from build123d import *

# Parameters (mm, degrees)
F1_DEPTH = 92.5
F2_W     = 220
F2_H     = 175
F3_DEPTH = 200
F4_DEPTH = 195
F5_DEPTH = 2
F6_DEPTH = 2


with BuildPart() as f1:
    # F0 (on Front) → F1 (new body, symmetric)
    with BuildSketch(Plane.XZ):
        with BuildLine():
            Line((-39.8502688743, 141.3978409826), (-105.0004470674, 141.3978409826))
            Line((-105.0004470674, 141.3978409826), (-105.0004470674, -28.6021590174))
            Line((-105.0004470674, -28.6021590174), (124.9995529326, -28.6021590174))
            Line((124.9995529326, -28.6021590174), (124.9995529326, 51.3978409826))
            Line((124.9995529326, 51.3978409826), (0, 134.314134717))
            ThreePointArc((0, 134.314134717), (-19.6127861763, 139.6131417621), (-39.8502688743, 141.3978409826))
        make_face()
    extrude(amount=F1_DEPTH, both=True)

    # F2 (on face) → F3 (join)
    with BuildSketch(Plane(origin=(0, 0, -28.6021590174), x_dir=(1, 0, 0), z_dir=(0, 0, -1))):
        with Locations((9.9995529326, 0)):
            Rectangle(F2_W, F2_H)
    extrude(amount=-F3_DEPTH)

    # F4 (cut): a face of the model
    f4_faces = [f1.faces().sort_by_distance(p)[0] for p in [
        (9.9995529326, 0, 171.3978409826),
    ]]
    extrude(f4_faces, amount=-F4_DEPTH, mode=Mode.SUBTRACT)

    # F5 (add): a face of the model
    f5_faces = [f1.faces().sort_by_distance(p)[0] for p in [
        (-100.0004470674, 0, 58.8978409826),
    ]]
    extrude(f5_faces, amount=F5_DEPTH)

    # F6 (add): a face of the model
    f6_faces = [f1.faces().sort_by_distance(p)[0] for p in [
        (119.9995529326, 0, 15.5561727884),
    ]]
    extrude(f6_faces, amount=F6_DEPTH)


solid = f1.part
The listing builds one solid part. Answer for the finished solid, in the listing's coordinates (mm). A direction names the side the tool comes from. Give positions to 0.01 mm unless a question says otherwise; leave off trailing zeros. Write each loop counter-clockwise with the first axis right and the second up, starting at its lowest first coordinate (ties: lowest second). Pieces come first, ordered by that corner, then holes. Notation, with made-up numbers: (42, 48.25) - (69, 48.25) arc R27 cw to (69, 72.25) - close; hole circle Ø1 at (-19.5, 19). An arc over 180 degrees is marked (long way). Use a Markdown table: item, result.
1. Section A-A on z = 7 is taken. Write down the section's boundary in (x, y), plus the area to 3 significant figures.
Values follow:
| item | result |
|---|---|
| outline | (-105, -92.5) - (125, -92.5) - (125, 92.5) - (-105, 92.5) - close; hole (-98, -87.5) - (118, -87.5) - (118, 87.5) - (-98, 87.5) - close |
| area | 4,750 mm² |
2. Section C-C on y = -6.5 is taken. Write down the section's boundary in (x, z), plus the area to 3 significant figures.
Values follow:
| item | result |
|---|---|
| outline | (-105, -28.6) - (125, -28.6) - (125, 51.4) - (120, 54.71) - (118, 54.71) - (118, -23.6) - (-98, -23.6) - (-98, 141.4) - (-105, 141.4) - close |
| area | 2,840 mm² |
3. A tool of negligible diameter and unlimited length cuts with its end or side. For faces 1 (the flat face through (125, -1, 11)), 2 (the flat face through (8, -1, -23.602)), from which of +Z, -Z, +X, -X, +Y, -Y can it reach the whole face along a straight path? Write none if from no direction.
Values follow:
| item | result |
|---|---|
| face 1 | +Z, -Z, +X, +Y, -Y |
| face 2 | +Z |
4. Section D-D on z = 70 is taken. Write down the section's boundary in (x, y), plus the area to 3 significant figures.
Values follow:
| item | result |
|---|---|
| outline | (-105, -92.5) - (96.96, -92.5) - (96.96, -87.5) - (-98, -87.5) - (-98, 87.5) - (96.96, 87.5) - (96.96, 92.5) - (-105, 92.5) - close |
| area | 3,240 mm² |
5. Each of these flat-tipped pins is pushed along its axis until it touches: P1, Ø0.6, axis at x = 118.5, y = -26, coming from the +Z side; P2, Ø5, axis at x = -65, y = 28.5, coming from the +Z side. Where does it stop, or does it pass through?
Values follow:
| item | result |
|---|---|
| P1 | stops at z = 54.71 |
| P2 | stops at z = -23.6 |
6. For a pull along Y with two mould halves and no side action, classify faces 3 (the flat face through (9, 87.5, 42)), 4 (the flat face through (8, -92.5, 39)), 5 (the flat face through (8, -1, -28.602)) as released by +Y, released by -Y, zero draft, split by the parting line, or undercut.
Values follow:
| item | result |
|---|---|
| face 3 | undercut |
| face 4 | released by -Y |
| face 5 | zero draft |
7. Section B-B on x = -47 is taken. Write down the section's boundary in (y, z).
Values follow:
| item | result |
|---|---|
| outline | (-92.5, -28.6) - (92.5, -28.6) - (92.5, 141.4) - (87.5, 141.4) - (87.5, -23.6) - (-87.5, -23.6) - (-87.5, 141.4) - (-92.5, 141.4) - close |
8. Find the intervals of material crossed by probe 1 along Y at (x, z) = (37, 76); probe 2 along X at (y, z) = (-50, 35); probe 3 along X at (y, z) = (24.5, 128), in increasing order. Write a range as from..to.
Values follow:
| item | result |
|---|---|
| probe 1 | y = -92.5..-87.5, 87.5..92.5 |
| probe 2 | x = -105..-98, 118..125 |
| probe 3 | x = -105..-98 |
